```python
from build123d import *

# Parameters (mm, degrees)
F0_R     = 876.3
F0_R_2   = 50.8
F0_R_3   = 571.5
F1_DEPTH = 76.2
F0_R_4   = 527.05
F2_DEPTH = 406.4


# Not quite as in the source:
# - a feature names something its author has since deleted; it is built from what else it names


with BuildPart() as f1:
    # F0 (on Top) → F1 (new body)
    with BuildSketch(Plane.XY):
        Circle(F0_R)
        with Locations((0, -723.9)):
            Circle(F0_R_2, mode=Mode.SUBTRACT)
        with Locations((-723.9, 0)):
            Circle(F0_R_2, mode=Mode.SUBTRACT)
        Circle(F0_R_3, mode=Mode.SUBTRACT)
        with Locations((723.9, 0)):
            Circle(F0_R_2, mode=Mode.SUBTRACT)
        with Locations((0, 723.9)):
            Circle(F0_R_2, mode=Mode.SUBTRACT)
    extrude(amount=F1_DEPTH)

    # F0 (on Top) → F2 (join)
    with BuildSketch(Plane.XY):
        Circle(F0_R_3)
        Circle(F0_R_4, mode=Mode.SUBTRACT)
    extrude(amount=F2_DEPTH)


solid = f1.part
```
Part model, mm, in its own coordinate system. A direction names the side the tool comes from. Give positions to 0.01 mm unless a question says otherwise; leave off trailing zeros. Order: outer loops, then holes, each group sorted by start corner. A loop starts at its lowest first (then second) coordinate and runs counter-clockwise, first axis right, second up. Notation, with made-up numbers: M 81,-20.75 L 103,-20.75 A15 cw 103,7.25 Z; hole C 65.25,80 d5. An arc over 180 degrees is marked long. Use a Markdown table: item, result. Add a question column.
(1) Mould opens along X. For faces 1 (the face through (-11.012, -773.492, 37.567)), 2 (the face through (-570.947, 25.128, 238.989)), 3 (the face through (-388.458, 356.205, 200.355)), 4 (the face through (167, -505, 406.4)) say: +X half, -X half, draft (parallel to the pull), parting line (faces both ways), or undercut.
(2) Saw through at B-B, the plane x = 368. Give the cut face in (y, z), and give its area (3 significant figures).
(3) Saw through at A-A, the plane y = 0. Give the cut face in (x, z).
(4) Probe line 1 along Y through (x, z) = (0, 28); line 2 along Z through (x, y) = (-426, -722); line 3 along Y through (x, z) = (-216.5, 192). List the from-to ranges inside material, lowest first. Write a range as [from, to].
(5) 3-axis set-ups, long thin cutter, end or side, ignore diameter. For faces 5 (the face through (-12, -572, 76.2)), 6 (the face through (27.31, 766.735, 37.567)): which of +Z, -Z, +X, -X, +Y, -Y reach the whole face in a straight line?
(6) Drop flat-ended pins along their axis: P1, Ø4, axis at x = 71, z = 202.5, coming from the +Y side; P2, Ø1, axis at y = -236.5, z = 202.5, coming from the -X side; P3, Ø10, axis at x = 620, y = 92.5, coming from the +Z side. Give the stop position or say it passes through.
(7) Saw through at D-D, the plane z = 339.5. Give the cut face in (x, y), and give its area (3 significant figures).
Answer key:
| question | item | result |
|---|---|---|
| 1 | face 1 | undercut |
| 1 | face 2 | parting line |
| 1 | face 3 | undercut |
| 1 | face 4 | draft |
| 2 | outline | M -795.28,0 L -377.3,0 L -377.3,406.4 L -437.25,406.4 L -437.25,76.2 L -795.28,76.2 Z; M 377.3,0 L 795.28,0 L 795.28,76.2 L 437.25,76.2 L 437.25,406.4 L 377.3,406.4 Z |
| 2 | area | 103,000 mm^2 |
| 3 | outline | M -876.3,0 L -774.7,0 L -774.7,76.2 L -876.3,76.2 Z; M -673.1,0 L -527.05,0 L -527.05,406.4 L -571.5,406.4 L -571.5,76.2 L -673.1,76.2 Z; M 527.05,0 L 673.1,0 L 673.1,76.2 L 571.5,76.2 L 571.5,406.4 L 527.05,406.4 Z; M 774.7,0 L 876.3,0 L 876.3,76.2 L 774.7,76.2 Z |
| 4 | line 1 | [-876.3, -774.7], [-673.1, -527.05], [527.05, 673.1], [774.7, 876.3] |
| 4 | line 2 | [0, 76.2] |
| 4 | line 3 | [-528.9, -480.53], [480.53, 528.9] |
| 5 | face 5 | +Z |
| 5 | face 6 | +Z, -Z |
| 6 | P1 | y = 567.32 |
| 6 | P2 | x = -520.5 |
| 6 | P3 | z = 76.2 |
| 7 | outline | C 0,0 d1143; hole C 0,0 d1054.1 |
| 7 | area | 153,000 mm^2 |
